The listing builds one solid part. Answer for the finished solid, in the listing's coordinates (mm). Round coordinates to 2 decimals unless told otherwise and drop trailing zeros. Order: outer loops, then holes, each group sorted by start corner. A loop starts at its lowest first (then second) coordinate and runs counter-clockwise, first axis right, second up. Notation, with made-up numbers: (14, -38) - (54, -38) arc R15 cw to (54, -25) - close; hole circle Ø6 at (64, -1.5). An arc over 180 degrees is marked (long way). One line per item, written item: value. Start each with the question number.
1. Section C-C, the plane z = 8.75 is taken. Give the vertices of the cut face in (x, y).
2. Section A-A, the plane x = 7 is taken. Give the vertices of the cut face in (y, z).
3. Straight lines are drawn through the part: line 1 (X direction, y = 3.1, z = 16.25); line 2 (X direction, y = 4.5, z = 12); line 3 (Y direction, x = 5, z = 6.75). For each, find the intervals that lie inside material, in ascending order.
4. For a pull along Y with two mould halves and no side action, classify faces 1 (the flat face through (9, 0, 11)), 2 (the cylindrical face through (7.1, 6.1, 11.2)), 3 (the flat face through (7, 7, 0)), 4 (the cylindrical face through (7.66, 0.173, 11.154)) as released by +Y, released by -Y, zero draft, split by the parting line, or undercut.
5. Section B-B, the plane y = 3.1 is taken. Give the vertices of the cut face in (x, z).
6. A flat-ended cylindrical pin translates along its axis: P1, Ø1, axis at x = 7, y = 4, coming from the -Z side. Find the tip coordinate at first contact, or state that the pin passes through.
Autodesk Inventor part; units mm, degrees
ref_plane "YZ Plane" through (0, 0, 0) normal (1, 0, 0) x (0, 1, 0)
ref_plane "XZ Plane" through (0, 0, 0) normal (0, 1, 0) x (-1, 0, 0)
ref_plane "XY Plane" through (0, 0, 0) normal (0, 0, 1) x (1, 0, 0)
sketch "Szkic1" plane through (0, 0, 0) normal (0, 1, 0) x (-1, 0, 0)
  line L0 (0, 0) -> (-14, 0)
  line L1 (-14, 0) -> (-14, 22)
  line L2 (-14, 22) -> (0, 22)
  line L3 (0, 22) -> (0, 0)
  dimension "d0" = 14
  dimension "d1" = 22
extrude "Wyciągnięcie proste1" add sketch "Szkic1" along normal blind 8.25
sketch "Szkic2" plane through (0, 0, 22) normal (0, 0, 1) x (1, 0, 0)
  circle A0 centre (7, 3.1) radius 1
  arc A1 (8, 0.2716) -> (6, 0.2716) centre (7, 3.1) ccw
  line L0 (6, 0.2716) -> (6, 0)
  line L1 (6, 0) -> (8, 0)
  line L2 (8, 0) -> (8, 0.2716)
  circle A2 centre (7, 3.1) radius 3
  point P0 (0, 0)
  point P1 (6, 0.2716)
extrude "Wyciągnięcie proste2" cut sketch "Szkic2" against normal through all contours A0 | A2 A1
sketch "Szkic3" plane through (0, 8.25, 0) normal (0, 1, 0) x (1, 0, 0)
  line L0 (0, -22) -> (14, -22)
  line L1 (14, -22) -> (14, 0)
  line L2 (14, 0) -> (0, 0)
  line L3 (0, 0) -> (0, -22)
extrude "Wyciągnięcie proste3" add sketch "Szkic3" along normal blind 4
properties part number "uchwyt silnikow"
Answer list:
1. outline: (0, 0) - (14, 0) - (14, 12.25) - (0, 12.25) - close; hole circle Ø6 at (7, 3.1)
2. outline: (0, 0) - (0.1, 0) - (0.1, 22) - (0, 22) - close; (6.1, 0) - (12.25, 0) - (12.25, 22) - (6.1, 22) - close
3. line 1: x = 0 to 4, 10 to 14
3. line 2: x = 0 to 4.35, 9.65 to 14
3. line 3: y = 0 to 0.86, 5.34 to 12.25
4. face 1: released by -Y
4. face 2: undercut
4. face 3: zero draft
4. face 4: undercut
5. outline: (0, 0) - (4, 0) - (4, 22) - (0, 22) - close; (10, 0) - (14, 0) - (14, 22) - (10, 22) - close
6. P1: passes through
